Design review of the part built by this model. Coordinates are the model's own, in mm. Face numbers are marked on the shaded views. Coordinates: 2 decimals unless noted, no trailing zeros. Order: outer loops, then holes, each group sorted by start corner. A loop starts at its lowest first (then second) coordinate and runs counter-clockwise, first axis right, second up. Notation, with made-up numbers: M 8.25,-30.5 L 15.25,-30.5 A16 ccw 15.25,-1.5 Z; hole C 73.25,43 d6. An arc over 180 degrees is marked long. Answer as a JSON object with one key per item and string values.
from build123d import *

# Parameters (mm, degrees)
SKETCH1_W           = 513.08
SKETCH1_H           = 330.2
BOSS_EXTRUDE1_DEPTH = 50.8
SKETCH2_R           = 12.7
CUT_EXTRUDE1_DEPTH  = 331.2
SKETCH3_W           = 382.967058901
SKETCH3_H           = 19.05
BOSS_EXTRUDE2_DEPTH = 12.7
SKETCH4_W           = 383.722022032
SKETCH4_H           = 44.45
BOSS_EXTRUDE3_DEPTH = 12.7


with BuildPart() as part:
    # Sketch1 → Boss-Extrude1 (new body)
    with BuildSketch(Plane(origin=(0, 0, 0), x_dir=(1, 0, 0), z_dir=(0, 1, 0))):
        with Locations((28.712036474, 1.505471125)):
            Rectangle(SKETCH1_W, SKETCH1_H)
    extrude(amount=BOSS_EXTRUDE1_DEPTH)

    # Sketch2 → Cut-Extrude1 (cut, through all)
    with BuildSketch(Plane.XY.offset(163.594528875)):
        with Locations((-192.209486062, 24.51392069)):
            Circle(SKETCH2_R)
        Polygon((-151.627963526, 0), (285.252036474, 50.8), (285.252036474, 0), align=None)
    extrude(amount=-CUT_EXTRUDE1_DEPTH, mode=Mode.SUBTRACT)

    # Sketch3 → Boss-Extrude2 (add)
    with BuildSketch(Plane(origin=(-2.022784999, 17.395950991, 0), x_dir=(0.99330738, 0.115500858, 0), z_dir=(0.115500858, -0.99330738, 0))):
        with Locations((77.492959748, -131.680471125)):
            Rectangle(SKETCH3_W, SKETCH3_H)
    boss_extrude2 = extrude(amount=BOSS_EXTRUDE2_DEPTH)

    # Sketch4 → Boss-Extrude3 (add)
    with BuildSketch(Plane(origin=(-0.5559241, 4.780947262, 0), x_dir=(0.99330738, 0.115500858, 0), z_dir=(0.115500858, -0.99330738, 0))):
        with Locations((77.870441313, -131.680471125)):
            Rectangle(SKETCH4_W, SKETCH4_H)
    boss_extrude3 = extrude(amount=BOSS_EXTRUDE3_DEPTH)

    # Mirror1: Boss-Extrude2, Boss-Extrude3 across plane
    add(boss_extrude2.mirror(Plane.XY.offset(-1.505471125)))
    add(boss_extrude3.mirror(Plane.XY.offset(-1.505471125)))


solid = part.part
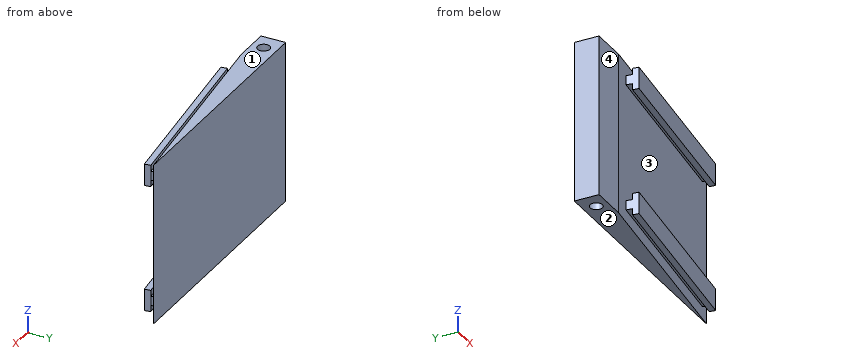
1) Insertion check: pin 1 Ø8 at (x, y) = (-51.5, 5.5) entering from +Z; pin 2 Ø17 at (x, y) = (116, 2) entering from +Z; pin 3 Ø2 at (x, z) = (-70, 14.5) entering from -Y. Each pin has a flat end and moves straight along its axis. Give the tip position at first contact, or say it passes through.
Taken from the geometry:
{"pin 1": "stops at z = 138.19", "pin 2": "stops at z = 150.89", "pin 3": "stops at y = 9.38"}
2) Add section D-D (z = -131.5). State the section outline as (x, y) points, and give its area (3 significant figures).
Taken from the geometry:
{"outline": "M -227.83,0 L -151.63,0 L -115.25,4.23 L -112.32,-21 L 268.84,23.32 L 267.37,35.94 L 266.62,35.85 L 265.15,48.46 L 285.25,50.8 L -227.83,50.8 Z; hole C -192.21,24.51 d25.4", "area": "24,200 mm2"}
3) Add section B-B (y = 17). State the section outline as (x, z) points.
Taken from the geometry:
{"outline": "M -227.83,-166.61 L -202.45,-166.61 L -202.45,163.59 L -227.83,163.59 Z; M -181.97,-166.61 L -5.43,-166.61 L -5.43,-141.21 L 104.53,-141.21 L 104.53,-153.91 L 214.48,-153.91 L 214.48,-109.46 L 104.53,-109.46 L 104.53,-122.16 L -5.43,-122.16 L -5.43,119.14 L 104.53,119.14 L 104.53,106.44 L 214.48,106.44 L 214.48,150.89 L 104.53,150.89 L 104.53,138.19 L -5.43,138.19 L -5.43,163.59 L -181.97,163.59 Z"}
4) Mouldability with a two-part tool opening along Z and no side actions: class the marked faces 1, 2, 3 and 4 as released by +Z, released by -Z, zero draft, split by the parting line, or undercut.
Taken from the geometry:
{"face 1": "released by +Z", "face 2": "released by -Z", "face 3": "undercut", "face 4": "zero draft"}
5) Add section C-C (x = 8.5). State the section outline as (y, z) points.
Taken from the geometry:
{"outline": "M -6.95,-153.91 L 5.83,-153.91 L 5.83,-141.21 L 18.62,-141.21 L 18.62,-166.61 L 50.8,-166.61 L 50.8,163.59 L 18.62,163.59 L 18.62,138.19 L 5.83,138.19 L 5.83,150.89 L -6.95,150.89 L -6.95,106.44 L 5.83,106.44 L 5.83,119.14 L 18.62,119.14 L 18.62,-122.16 L 5.83,-122.16 L 5.83,-109.46 L -6.95,-109.46 Z"}
6) Add section A-A (z = 113). State the section outline as (x, y) points, and give its area (3 significant figures).
Taken from the geometry:
{"outline": "M -227.83,0 L -151.63,0 L 285.25,50.8 L -227.83,50.8 Z; M -113.78,-8.39 L -112.32,-21 L 268.84,23.32 L 267.37,35.94 Z; hole C -192.21,24.51 d25.4", "area": "19,300 mm2"}
7) To check wall thickness, follow L1, parallel to Z at x = -87.5, y = 3; L2, parallel to Z at x = 181.5, y = 22; L3, parallel to Y at x = -192, z = -143. State the ranges of each line that lie inside material, in increasing order.
Taken from the geometry:
{"L1": "z = -141.21 to -122.16, 119.14 to 138.19", "L2": "z = -153.91 to -109.46, 106.44 to 150.89", "L3": "y = 0 to 11.82, 37.21 to 50.8"}
